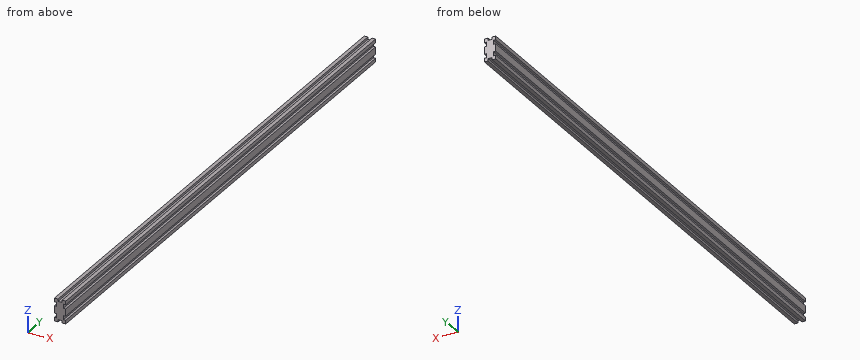
Solid Edge part; units mm, degrees
sketch "Sketch1" plane through (0, 0, 0) normal (0, -1, 0) x (1, 0, 0)
  line L0 (12.7, -25.4) -> (12.7, -17.3179)
  line L1 (12.7, -17.3179) -> (7.62, -17.3179)
  line L2 (7.62, -17.3179) -> (7.62, -8.0821)
  line L3 (7.62, -8.0821) -> (12.7, -8.0821)
  line L4 (12.7, -8.0821) -> (12.7, 0)
  line L5 (12.7, 8.0821) -> (12.7, 0)
  line L6 (7.62, 8.0821) -> (12.7, 8.0821)
  line L7 (7.62, 17.3179) -> (7.62, 8.0821)
  line L8 (12.7, 17.3179) -> (7.62, 17.3179)
  line L9 (12.7, 25.4) -> (12.7, 17.3179)
  line L10 (4.6179, 25.4) -> (12.7, 25.4)
  line L11 (4.6179, 25.4) -> (4.6179, 20.32)
  line L12 (4.6179, 20.32) -> (-4.6179, 20.32)
  line L13 (-4.6179, 20.32) -> (-4.6179, 25.4)
  line L14 (-12.7, 25.4) -> (-4.6179, 25.4)
  line L15 (-12.7, 17.3179) -> (-12.7, 25.4)
  line L16 (-7.62, 17.3179) -> (-12.7, 17.3179)
  line L17 (-7.62, 8.0821) -> (-7.62, 17.3179)
  line L18 (-12.7, 8.0821) -> (-7.62, 8.0821)
  line L19 (-12.7, 0) -> (-12.7, 8.0821)
  line L20 (-12.7, 0) -> (-12.7, -8.0821)
  line L21 (-12.7, -8.0821) -> (-7.62, -8.0821)
  line L22 (-7.62, -8.0821) -> (-7.62, -17.3179)
  line L23 (-7.62, -17.3179) -> (-12.7, -17.3179)
  line L24 (-12.7, -17.3179) -> (-12.7, -25.4)
  line L25 (-12.7, -25.4) -> (-4.6179, -25.4)
  line L26 (-4.6179, -20.32) -> (-4.6179, -25.4)
  line L27 (4.6179, -20.32) -> (-4.6179, -20.32)
  line L28 (4.6179, -25.4) -> (4.6179, -20.32)
  line L29 (4.6179, -25.4) -> (12.7, -25.4)
extrude "Protrusion1" add sketch "Sketch1" against normal blind 1219.2
Input: part model. Units: mm. Frame: model coordinates. Give positions to 0.01 mm unless a question says otherwise; leave off trailing zeros. Order: outer loops, then holes, each group sorted by start corner. A loop starts at its lowest first (then second) coordinate and runs counter-clockwise, first axis right, second up. Notation, with made-up numbers: (-38.5, 53.5) - (5.5, 53.5) arc R22 ccw to (5.5, 72.5) - close; hole circle Ø5 at (26, 40). An arc over 180 degrees is marked (long way). Put each result on its own line as item: value.
Item 1: Ray query, L1, parallel to Z at x = -10.75, y = 173; L2, parallel to X at y = 136.5, z = 21; L3, parallel to Z at x = -0.5, y = 725.5. Return the intervals inside material, ascending. Write a range as from..to.
Found:
L1: z = -25.4..-17.32, -8.08..8.08, 17.32..25.4
L2: x = -12.7..-4.62, 4.62..12.7
L3: z = -20.32..20.32
Item 2: Contact query for flat-ended pins moving along their axis: pin 1 (3 mm diameter, centred on y = 609.5, z = 12.5, fed in from -X); pin 2 (3 mm diameter, centred on y = 652, z = 13.5, fed in from +X); pin 3 (4.5 mm diameter, centred on x = 1.5, y = 527.5, fed in from +Z). Output: stop coordinate, or through.
Found:
pin 1: stops at x = -7.62
pin 2: stops at x = 7.62
pin 3: stops at z = 20.32
Item 3: Section query A-A, the plane y = 1073.5. Return loops of the section in (x, z), then the cut area to 3 significant figures.
Found:
outline: (-12.7, -25.4) - (-4.62, -25.4) - (-4.62, -20.32) - (4.62, -20.32) - (4.62, -25.4) - (12.7, -25.4) - (12.7, -17.32) - (7.62, -17.32) - (7.62, -8.08) - (12.7, -8.08) - (12.7, 8.08) - (7.62, 8.08) - (7.62, 17.32) - (12.7, 17.32) - (12.7, 25.4) - (4.62, 25.4) - (4.62, 20.32) - (-4.62, 20.32) - (-4.62, 25.4) - (-12.7, 25.4) - (-12.7, 17.32) - (-7.62, 17.32) - (-7.62, 8.08) - (-12.7, 8.08) - (-12.7, -8.08) - (-7.62, -8.08) - (-7.62, -17.32) - (-12.7, -17.32) - close
area: 1,010 mm^2
